from build123d import *

# Parameters (mm, degrees)
F1_DEPTH    = 21
F2_R        = 10.5
F3_DEPTH    = 25
F4_T1_DEPTH = 30.3938312155


# Not quite as in the source:
# - a fillet or chamfer that OpenCascade refuses, or shapes differently, is made with other operations: its cross-section is extruded or revolved along the edge and cut away or added


with BuildPart() as f1:
    # F0 (on Right) → F1 (new body)
    with BuildSketch(Plane.YZ):
        Polygon((-135, -5), (135, -45), (135, 25), (-135, 25), align=None)
    extrude(amount=F1_DEPTH)

    # F2 (on face) → F3 (cut)
    with BuildSketch(Plane.YZ.offset(21)):
        with Locations((110, 21)):
            Circle(F2_R)
        with Locations((56, 21)):
            Circle(F2_R)
        with Locations((2, 21)):
            Circle(F2_R)
        with Locations((-52, 21)):
            Circle(F2_R)
        with Locations((-106, 21)):
            Circle(F2_R)
    extrude(amount=-F3_DEPTH, mode=Mode.SUBTRACT)

    # F4: chamfer of 2 on 10 edges, made by hand

    # F4_s2 → F4_t1 (cut)
    with BuildSketch(Plane.YZ.offset(-4.6969156077)):
        with BuildLine():
            Line((-117.5859668407, 25.062603733), (-116.1815447498, 23.2973611197))
            Line((-116.1815447498, 23.2973611197), (-116.1425681704, 23.2883707774))
            ThreePointArc((-116.1425681704, 23.2883707774), (-115.9721143456, 24.157298763), (-115.6712601331, 24.9847619048))
            Line((-115.6712601331, 24.9847619048), (-115.7082439195, 25.04))
            ThreePointArc((-115.7082439195, 25.04), (-116.6471053801, 25.04), (-117.5859668407, 25.102603733))
            Line((-117.5859668407, 25.102603733), (-117.5859668407, 25.062603733))
        make_face()
        with BuildLine():
            Line((-95.8184552502, 23.2973611197), (-94.4140331593, 25.062603733))
            Line((-94.4140331593, 25.062603733), (-94.4140331593, 25.102603733))
            ThreePointArc((-94.4140331593, 25.102603733), (-95.3528946199, 25.04), (-96.2917560805, 25.04))
            Line((-96.2917560805, 25.04), (-96.3287398669, 24.9847619048))
            ThreePointArc((-96.3287398669, 24.9847619048), (-96.0278856544, 24.157298763), (-95.8574318296, 23.2883707774))
            Line((-95.8574318296, 23.2883707774), (-95.8184552502, 23.2973611197))
        make_face()
        with BuildLine():
            Line((-63.5859668407, 25.062603733), (-62.1815447498, 23.2973611197))
            Line((-62.1815447498, 23.2973611197), (-62.1425681704, 23.2883707774))
            ThreePointArc((-62.1425681704, 23.2883707774), (-61.9721143456, 24.157298763), (-61.6712601331, 24.9847619048))
            Line((-61.6712601331, 24.9847619048), (-61.7082439195, 25.04))
            ThreePointArc((-61.7082439195, 25.04), (-62.6471053801, 25.04), (-63.5859668407, 25.102603733))
            Line((-63.5859668407, 25.102603733), (-63.5859668407, 25.062603733))
        make_face()
        with BuildLine():
            Line((-41.8184552502, 23.2973611197), (-40.4140331593, 25.062603733))
            Line((-40.4140331593, 25.062603733), (-40.4140331593, 25.102603733))
            ThreePointArc((-40.4140331593, 25.102603733), (-41.3528946199, 25.04), (-42.2917560805, 25.04))
            Line((-42.2917560805, 25.04), (-42.3287398669, 24.9847619048))
            ThreePointArc((-42.3287398669, 24.9847619048), (-42.0278856544, 24.157298763), (-41.8574318296, 23.2883707774))
            Line((-41.8574318296, 23.2883707774), (-41.8184552502, 23.2973611197))
        make_face()
        with BuildLine():
            Line((-9.5859668407, 25.062603733), (-8.1815447498, 23.2973611197))
            Line((-8.1815447498, 23.2973611197), (-8.1425681704, 23.2883707774))
            ThreePointArc((-8.1425681704, 23.2883707774), (-7.9721143456, 24.157298763), (-7.6712601331, 24.9847619048))
            Line((-7.6712601331, 24.9847619048), (-7.7082439195, 25.04))
            ThreePointArc((-7.7082439195, 25.04), (-8.6471053801, 25.04), (-9.5859668407, 25.102603733))
            Line((-9.5859668407, 25.102603733), (-9.5859668407, 25.062603733))
        make_face()
        with BuildLine():
            Line((12.1815447498, 23.2973611197), (13.5859668407, 25.062603733))
            Line((13.5859668407, 25.062603733), (13.5859668407, 25.102603733))
            ThreePointArc((13.5859668407, 25.102603733), (12.6471053801, 25.04), (11.7082439195, 25.04))
            Line((11.7082439195, 25.04), (11.6712601331, 24.9847619048))
            ThreePointArc((11.6712601331, 24.9847619048), (11.9721143456, 24.157298763), (12.1425681704, 23.2883707774))
            Line((12.1425681704, 23.2883707774), (12.1815447498, 23.2973611197))
        make_face()
        with BuildLine():
            Line((44.4140331593, 25.062603733), (45.8184552502, 23.2973611197))
            Line((45.8184552502, 23.2973611197), (45.8574318296, 23.2883707774))
            ThreePointArc((45.8574318296, 23.2883707774), (46.0278856544, 24.157298763), (46.3287398669, 24.9847619048))
            Line((46.3287398669, 24.9847619048), (46.2917560805, 25.04))
            ThreePointArc((46.2917560805, 25.04), (45.3528946199, 25.04), (44.4140331593, 25.102603733))
            Line((44.4140331593, 25.102603733), (44.4140331593, 25.062603733))
        make_face()
        with BuildLine():
            Line((66.1815447498, 23.2973611197), (67.5859668407, 25.062603733))
            Line((67.5859668407, 25.062603733), (67.5859668407, 25.102603733))
            ThreePointArc((67.5859668407, 25.102603733), (66.6471053801, 25.04), (65.7082439195, 25.04))
            Line((65.7082439195, 25.04), (65.6712601331, 24.9847619048))
            ThreePointArc((65.6712601331, 24.9847619048), (65.9721143456, 24.157298763), (66.1425681704, 23.2883707774))
            Line((66.1425681704, 23.2883707774), (66.1815447498, 23.2973611197))
        make_face()
        with BuildLine():
            Line((98.4140331593, 25.062603733), (99.8184552502, 23.2973611197))
            Line((99.8184552502, 23.2973611197), (99.8574318296, 23.2883707774))
            ThreePointArc((99.8574318296, 23.2883707774), (100.0278856544, 24.157298763), (100.3287398669, 24.9847619048))
            Line((100.3287398669, 24.9847619048), (100.2917560805, 25.04))
            ThreePointArc((100.2917560805, 25.04), (99.3528946199, 25.04), (98.4140331593, 25.102603733))
            Line((98.4140331593, 25.102603733), (98.4140331593, 25.062603733))
        make_face()
        with BuildLine():
            Line((120.1815447498, 23.2973611197), (121.5859668407, 25.062603733))
            Line((121.5859668407, 25.062603733), (121.5859668407, 25.102603733))
            ThreePointArc((121.5859668407, 25.102603733), (120.6471053801, 25.04), (119.7082439195, 25.04))
            Line((119.7082439195, 25.04), (119.6712601331, 24.9847619048))
            ThreePointArc((119.6712601331, 24.9847619048), (119.9721143456, 24.157298763), (120.1425681704, 23.2883707774))
            Line((120.1425681704, 23.2883707774), (120.1815447498, 23.2973611197))
        make_face()
    extrude(amount=F4_T1_DEPTH, mode=Mode.SUBTRACT)


solid = f1.part
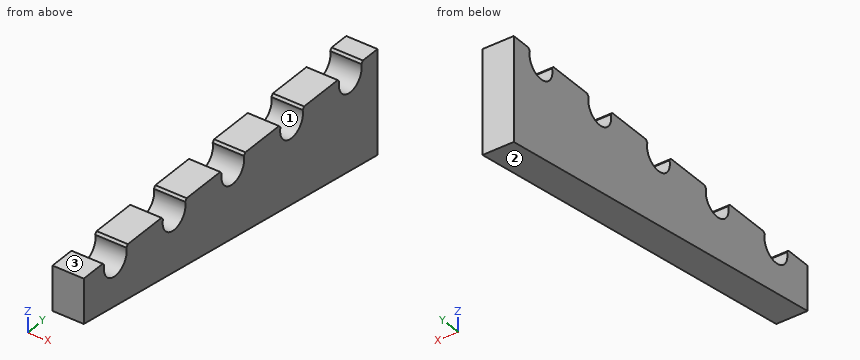
The model under review builds one solid part; all positions refer to its coordinate system, in mm. Face numbers are marked on the shaded views. Round coordinates to 2 decimals unless told otherwise and drop trailing zeros. Write each loop counter-clockwise with the first axis right and the second up, starting at its lowest first coordinate (ties: lowest second). Pieces come first, ordered by that corner, then holes. Notation, with made-up numbers: (58, 75) - (111, 75) arc R27 cw to (111, 104) - close; hole circle Ø10 at (-4, 55.5). An arc over 180 degrees is marked (long way). One line per item, written item: value. Start each with the question number.
1. To check wall thickness, follow L1, parallel to Y at x = 13.5, z = 21; L2, parallel to Y at x = 13.75, z = 18; L3, parallel to Z at x = 7.5, y = 88. State the ranges of each line that lie inside material, in increasing order. Write a range as from..to.
2. Clearance check with flat-ended pins moving along their axes: P1, Ø24, axis at y = -52, z = 21, coming from the +X side; P2, Ø3, axis at x = 9.5, y = 87.5, coming from the -Z side; P3, Ø12.5, axis at y = 2, z = 21, coming from the +X side. State where each tip first meets the part, or that it passes through.
3. Consider section D-D on y = -57.5. Write out the cut boundary in (x, z).
4. The part is to be moulded in two halves that separate along Z. For the marked faces 1, 2 and 3, say which applies: released by +Z, released by -Z, zero draft, split by the parting line, or undercut.
5. Consider section C-C on z = -24. Write out the cut boundary in (x, y), and give its area (3 significant figures).
6. Consider section A-A on z = 21. Write out the cut boundary in (x, y), and give its area (4 significant figures).
7. Consider section B-B on x = 11.25. Write out the cut boundary in (y, z), and give its area (3 significant figures).
Checks:
1. L1: y = -135..-116.5, -95.5..-62.5, -41.5..-8.5, 12.5..45.5, 66.5..99.5, 120.5..135
1. L2: y = -135..-116.06, -95.94..-62.06, -41.94..-8.06, 12.06..45.94, 66.06..99.94, 120.06..135
1. L3: z = -38.04..25
2. P1: stops at x = 21
2. P2: stops at z = -38.19
2. P3: passes through
3. outline: (0, -16.48) - (21, -16.48) - (21, 12.06) - (0, 12.06) - close
4. face 1: undercut
4. face 2: released by -Z
4. face 3: released by +Z
5. outline: (0, -6.75) - (21, -6.75) - (21, 135) - (0, 135) - close
5. area: 2,980 mm^2
6. outline: (0, -135) - (21, -135) - (21, -116.5) - (0, -116.5) - close; (0, -95.5) - (21, -95.5) - (21, -62.5) - (0, -62.5) - close; (0, -41.5) - (21, -41.5) - (21, -8.5) - (0, -8.5) - close; (0, 12.5) - (21, 12.5) - (21, 45.5) - (0, 45.5) - close; (0, 66.5) - (21, 66.5) - (21, 99.5) - (0, 99.5) - close; (0, 120.5) - (21, 120.5) - (21, 135) - (0, 135) - close
6. area: 3,465 mm^2
7. outline: (-135, -5) - (135, -45) - (135, 25) - (121.54, 25) - (120.23, 23.36) arc R10.5 cw (long way) to (99.77, 23.36) - (98.46, 25) - (67.54, 25) - (66.23, 23.36) arc R10.5 cw (long way) to (45.77, 23.36) - (44.46, 25) - (13.54, 25) - (12.23, 23.36) arc R10.5 cw (long way) to (-8.23, 23.36) - (-9.54, 25) - (-40.46, 25) - (-41.77, 23.36) arc R10.5 cw (long way) to (-62.23, 23.36) - (-63.54, 25) - (-94.46, 25) - (-95.77, 23.36) arc R10.5 cw (long way) to (-116.23, 23.36) - (-117.54, 25) - (-135, 25) - close
7. area: 12,200 mm^2
